CAD build for the part. Positions are in the model's coordinates, mm. Face numbers are marked on the shaded views. A direction names the side the tool comes from. Round coordinates to 2 decimals unless told otherwise and drop trailing zeros. Loops run counter-clockwise (first coordinate to the right, second up) from the corner with the lowest first, then second, coordinate; pieces in that order, holes last. Notation, with made-up numbers: M 13.25,-22 L 71.25,-22 A21 ccw 71.25,10 Z; hole C -23.5,56 d10. An arc over 180 degrees is marked long. Use a Markdown table: item, result. Add a question column.
(1) Flat gauge pins, fed straight in: P1, Ø3, axis at x = -1, y = 17, coming from the +Z side; P2, Ø1, axis at x = -7.5, y = 29, coming from the +Z side; P3, Ø6, axis at x = -5, y = -8, coming from the -Z side. Where does each tip first touch, or does it go through?
(2) Band-saw the part on C-C, the plane z = 14. Write the cut outline in (x, y) (3 decimals), and give its area (3 significant figures).
(3) Which spindle directions (+Z, -Z, +X, -X, +Y, -Y) get a long thin tool onto all of the face, cutting with end or side? Do the marked faces 5, 6, 7, 8 and 9. Say none if no direction does.
(4) Band-saw the part on D-D, the plane y = 9. Write the cut outline in (x, z).
(5) Two-plate mould, pull along Z, no slides. Class the marked faces 1, 2, 3 and 4: released by +Z, released by -Z, zero draft, split by the parting line, or undercut.
(6) Band-saw the part on A-A, the plane x = -0.75. Write the cut outline in (y, z) (3 decimals), and give its area (3 significant figures).
(7) Band-saw the part on B-B, the plane y = 33. Write the cut outline in (x, z) (3 decimals), and give its area (3 significant figures).
(8) Wall check: L1, parallel to Y at x = -0.75, z = -3.65 (3 decimals); L2, parallel to Y at x = -5.75, z = 18 (3 decimals); L3, parallel to Z at x = -2.25, y = 6. Give the ranges that are in metal, low to high.
from build123d import *

# Parameters (mm, degrees)
BOSS_EXTRUDE1_DEPTH = 25
SKETCH2_R           = 1.5
CUT_EXTRUDE1_DEPTH  = 100
BOSS_EXTRUDE2_DEPTH = 6
CUT_EXTRUDE2_DEPTH  = 6
CUT_EXTRUDE3_DEPTH  = 6
SKETCH6_R           = 2
CUT_EXTRUDE4_DEPTH  = 60


with BuildPart() as part:
    # Sketch1 → Boss-Extrude1 (new body)
    with BuildSketch(Plane(origin=(0, 0, 0), x_dir=(1, 0, 0), z_dir=(0, 1, 0))):
        Polygon((-3, 3), (3, 3), (3, 4), (-4, 4), (-4, -4), (3, -4), (3, -3), (-3, -3), align=None)
    extrude(amount=BOSS_EXTRUDE1_DEPTH)

    # Sketch2 → Cut-Extrude1 (cut)
    with BuildSketch(Plane.XY.offset(4)):
        with Locations((-0.75, 3.105)):
            Circle(SKETCH2_R)
        with Locations((-0.75, 21.895)):
            Circle(SKETCH2_R)
    extrude(amount=-CUT_EXTRUDE1_DEPTH, mode=Mode.SUBTRACT)

    # Sketch3 → Boss-Extrude2 (add)
    with BuildSketch(Plane.ZY.offset(4)):
        with BuildLine():
            Line((-0.5, 42.5), (0.5, 42.5))
            ThreePointArc((0.5, 42.5), (1.914213562, 41.914213562), (2.5, 40.5))
            Line((2.5, 40.5), (2.5, 30))
            ThreePointArc((2.5, 30), (6.893398282, 19.393398282), (17.5, 15))
            Line((17.5, 15), (28, 15))
            ThreePointArc((28, 15), (29.414213562, 14.414213562), (30, 13))
            Line((30, 13), (30, 12))
            ThreePointArc((30, 12), (29.414213562, 10.585786438), (28, 10))
            Line((28, 10), (17.5, 10))
            ThreePointArc((17.5, 10), (6.893398282, 5.606601718), (2.5, -5))
            Line((2.5, -5), (2.5, -15.5))
            ThreePointArc((2.5, -15.5), (1.914213562, -16.914213562), (0.5, -17.5))
            Line((0.5, -17.5), (-0.5, -17.5))
            ThreePointArc((-0.5, -17.5), (-1.914213562, -16.914213562), (-2.5, -15.5))
            Line((-2.5, -15.5), (-2.5, -5))
            ThreePointArc((-2.5, -5), (-6.893398282, 5.606601718), (-17.5, 10))
            Line((-17.5, 10), (-28, 10))
            ThreePointArc((-28, 10), (-29.414213562, 10.585786438), (-30, 12))
            Line((-30, 12), (-30, 13))
            ThreePointArc((-30, 13), (-29.414213562, 14.414213562), (-28, 15))
            Line((-28, 15), (-17.5, 15))
            ThreePointArc((-17.5, 15), (-6.893398282, 19.393398282), (-2.5, 30))
            Line((-2.5, 30), (-2.5, 40.5))
            ThreePointArc((-2.5, 40.5), (-1.914213562, 41.914213562), (-0.5, 42.5))
        make_face()
        with BuildLine():
            Line((-27.312785606, 14.025), (-8.987997416, 14.025))
            ThreePointArc((-8.987997416, 14.025), (-7.462997416, 12.5), (-8.987997416, 10.975))
            Line((-8.987997416, 10.975), (-27.312785606, 10.975))
            ThreePointArc((-27.312785606, 10.975), (-28.837785606, 12.5), (-27.312785606, 14.025))
        make_face(mode=Mode.SUBTRACT)
        with BuildLine():
            Line((27.312785606, 14.025), (8.987997416, 14.025))
            ThreePointArc((8.987997416, 14.025), (7.462997416, 12.5), (8.987997416, 10.975))
            Line((8.987997416, 10.975), (27.312785606, 10.975))
            ThreePointArc((27.312785606, 10.975), (28.837785606, 12.5), (27.312785606, 14.025))
        make_face(mode=Mode.SUBTRACT)
        with BuildLine():
            Line((-1.525, -14.812785606), (-1.525, 3.512002584))
            ThreePointArc((-1.525, 3.512002584), (0, 5.037002584), (1.525, 3.512002584))
            Line((1.525, 3.512002584), (1.525, -14.812785606))
            ThreePointArc((1.525, -14.812785606), (0, -16.337785606), (-1.525, -14.812785606))
        make_face(mode=Mode.SUBTRACT)
        with BuildLine():
            Line((-1.525, 39.812785606), (-1.525, 21.487997416))
            ThreePointArc((-1.525, 21.487997416), (0, 19.962997416), (1.525, 21.487997416))
            Line((1.525, 21.487997416), (1.525, 39.812785606))
            ThreePointArc((1.525, 39.812785606), (0, 41.337785606), (-1.525, 39.812785606))
        make_face(mode=Mode.SUBTRACT)
    extrude(amount=BOSS_EXTRUDE2_DEPTH)

    # Sketch3_4 → Cut-Extrude2 (cut)
    with BuildSketch(Plane.ZY.offset(4)):
        with BuildLine():
            Line((-1.525, -14.812785606), (-1.525, 3.512002584))
            ThreePointArc((-1.525, 3.512002584), (0, 5.037002584), (1.525, 3.512002584))
            Line((1.525, 3.512002584), (1.525, -14.812785606))
            ThreePointArc((1.525, -14.812785606), (0, -16.337785606), (-1.525, -14.812785606))
        make_face()
    extrude(amount=-CUT_EXTRUDE2_DEPTH, mode=Mode.SUBTRACT)

    # Sketch3_5 → Cut-Extrude3 (cut)
    with BuildSketch(Plane.ZY.offset(4)):
        with BuildLine():
            Line((-1.525, 39.812785606), (-1.525, 21.487997416))
            ThreePointArc((-1.525, 21.487997416), (0, 19.962997416), (1.525, 21.487997416))
            Line((1.525, 21.487997416), (1.525, 39.812785606))
            ThreePointArc((1.525, 39.812785606), (0, 41.337785606), (-1.525, 39.812785606))
        make_face()
    extrude(amount=-CUT_EXTRUDE3_DEPTH, mode=Mode.SUBTRACT)

    # Sketch6 → Cut-Extrude4 (cut)
    with BuildSketch(Plane.ZY.offset(10)):
        with Locations((0, 12.5)):
            Circle(SKETCH6_R)
    extrude(amount=-CUT_EXTRUDE4_DEPTH, mode=Mode.SUBTRACT)


solid = part.part
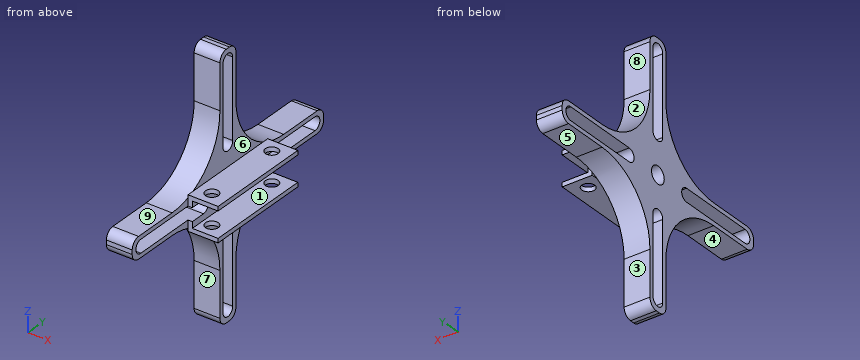
Return value:
| question | item | result |
|---|---|---|
| 1 | P1 | z = 4 |
| 1 | P2 | z = 2.58 |
| 1 | P3 | z = -2.5 |
| 2 | outline | M -10,9.586 L -4,9.586 L -4,10.975 L -10,10.975 Z; M -10,14.025 L -4,14.025 L -4,15.414 L -10,15.414 Z |
| 2 | area | 16.7 mm^2 |
| 3 | face 5 | -Z, +X, -X, +Y |
| 3 | face 6 | +Z, +X, +Y, -Y |
| 3 | face 7 | -Z, +X, -X, -Y |
| 3 | face 8 | +Z, +X, -X, +Y |
| 3 | face 9 | +Z, +X, -X, -Y |
| 4 | outline | M -10,-12.11 L -4,-12.11 L -4,-4 L 3,-4 L 3,-3 L -3,-3 L -3,3 L 3,3 L 3,4 L -4,4 L -4,12.11 L -10,12.11 Z |
| 5 | face 1 | undercut |
| 5 | face 2 | released by +Z |
| 5 | face 3 | zero draft |
| 5 | face 4 | released by -Z |
| 6 | outline | M 0,-4 L 1.605,-4 L 1.605,-3 L 0,-3 Z; M 0,3 L 1.605,3 L 1.605,4 L 0,4 Z; M 4.605,-4 L 20.395,-4 L 20.395,-3 L 4.605,-3 Z; M 4.605,3 L 20.395,3 L 20.395,4 L 4.605,4 Z; M 23.395,-4 L 25,-4 L 25,-3 L 23.395,-3 Z; M 23.395,3 L 25,3 L 25,4 L 23.395,4 Z |
| 6 | area | 38.0 mm^2 |
| 7 | outline | M -10,-2.5 L -4,-2.5 L -4,-1.525 L -10,-1.525 Z; M -10,1.525 L -4,1.525 L -4,2.5 L -10,2.5 Z |
| 7 | area | 11.7 mm^2 |
| 8 | L1 | 0 to 1.605, 4.605 to 20.395, 23.395 to 25 |
| 8 | L2 | 10 to 10.975, 14.025 to 15 |
| 8 | L3 | -4 to -3, 3 to 4 |
